The listing builds one solid part. Answer for the finished solid, in the listing's coordinates (mm). A direction names the side the tool comes from. Coordinates: 2 decimals unless noted, no trailing zeros. Order: outer loops, then holes, each group sorted by start corner. A loop starts at its lowest first (then second) coordinate and runs counter-clockwise, first axis right, second up. Notation, with made-up numbers: (39.25, 12) -> (57.25, 12) arc R28 ccw to (57.25, 49) -> close; hole circle Ø4 at (29.25, 79.5). An arc over 180 degrees is marked (long way). Write each question's results on one line, items separated by ' | '. Start each with the question number.
(1) A tool of negligible diameter and unlimited length cuts with its end or side. For faces 1 (the face through (6.897, 25.222, 10.819)), 2 (the face through (0, 38.1, 0)), 3 (the face through (6.897, -25.578, 10.819)), from which of +Z, -Z, +X, -X, +Y, -Y can it reach the whole face along a straight path? Write none if from no direction.
(2) Given pin 1 (2 mm diameter, centred on y = -12, z = 33, fed in from +X); pin 2 (3 mm diameter, centred on x = -12.5, z = 14, fed in from +Y); pin 3 (8 mm diameter, centred on y = 15, z = 30, fed in from -X), each flat-ended and moving along its own axis, determine where each tip first touches the part or whether it passes through.
(3) The part is cut by section B-B, the plane z = -8.5. Give the vertices of the cut face in (x, y).
(4) Straight lines are drawn through the part: L1, parallel to Y at x = 20.5, z = 13; L2, parallel to Y at x = -5.5, z = -4; L3, parallel to Z at x = 4, y = -13. For each, find the intervals that lie inside material, in ascending order.
(5) Determine the mould class of faces 4 (the face through (0, -38.1, 0)), 5 (the face through (0, -32, 25.682)), 6 (the face through (0, 0, -25.682)) for opening direction Z: +Z half, -Z half, draft (parallel to the pull), parting line (faces both ways), or undercut.
(6) The part is cut by section A-A, the plane z = 0. Give the vertices of the cut face in (x, y), then the cut area to 3 significant figures.
```python
from build123d import *

# Parameters (mm, degrees)
F0_W     = 63.627512
F0_H     = 51.364652
F0_R     = 12.830252
F1_DEPTH = 12.7
F2_DEPTH = 50.8
F3_DEPTH = 38.1


with BuildPart() as f1:
    # F0 (on Front) → F1 (new body, symmetric)
    with BuildSketch(Plane.XZ):
        Rectangle(F0_W, F0_H)
        Circle(F0_R, mode=Mode.SUBTRACT)
    extrude(amount=F1_DEPTH, both=True)

    # F0 (on Front) → F2 (join, symmetric)
    with BuildSketch(Plane.XZ):
        with BuildLine():
            Line((-31.813756, 25.682326), (31.813756, 25.682326))
            add(Edge.make_bspline(
                [(-31.813756, 25.682326), (-11.520594, 48.300739), (22.089949, 42.593289), (31.813756, 25.682326)],
                knots=[0, 0, 0, 0, 63.627511, 63.627511, 63.627511, 63.627511], degree=3))
        make_face()
    extrude(amount=F2_DEPTH, both=True)

    # F0 (on Front) → F3 (join, symmetric)
    with BuildSketch(Plane.XZ):
        Circle(F0_R)
    extrude(amount=F3_DEPTH, both=True)


solid = f1.part
```
Established:
1) face 1: +Y | face 2: -Z, +X, -X, +Y | face 3: -Y
2) pin 1: stops at x = 26.52 | pin 2: stops at y = 12.7 | pin 3: stops at x = -31.53
3) outline: (-31.81, -12.7) -> (-9.61, -12.7) -> (-9.61, -38.1) -> (9.61, -38.1) -> (9.61, -12.7) -> (31.81, -12.7) -> (31.81, 12.7) -> (9.61, 12.7) -> (9.61, 38.1) -> (-9.61, 38.1) -> (-9.61, 12.7) -> (-31.81, 12.7) -> close
4) L1: y = -12.7 to 12.7 | L2: y = -38.1 to 38.1 | L3: z = -12.19 to 12.19, 25.68 to 40.5
5) face 4: draft | face 5: undercut | face 6: -Z half
6) outline: (-31.81, -12.7) -> (-12.83, -12.7) -> (-12.83, -38.1) -> (12.83, -38.1) -> (12.83, -12.7) -> (31.81, -12.7) -> (31.81, 12.7) -> (12.83, 12.7) -> (12.83, 38.1) -> (-12.83, 38.1) -> (-12.83, 12.7) -> (-31.81, 12.7) -> close | area: 2,920 mm^2
